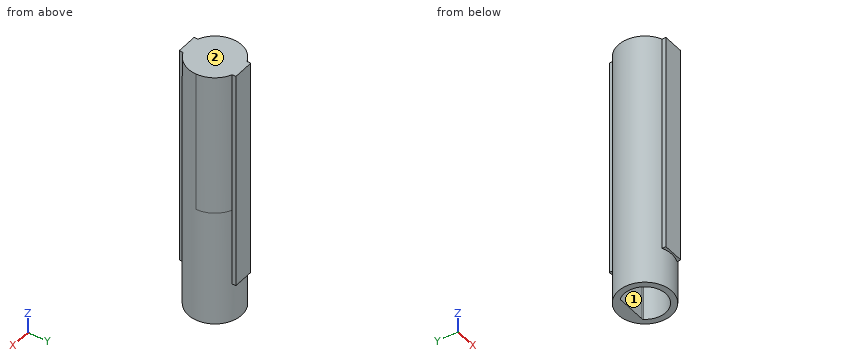
from build123d import *
from build123d.topology import SkipClean

# Parameters (mm, degrees)
SKETCH1_R                = 2
BOSS_EXTRUDE1_DEPTH      = 7
SKETCH3_R                = 2
SKETCH3_W                = 4.25
SKETCH3_H                = 1.5
BOSS_EXTRUDE3_DEPTH      = 4
BOSS_EXTRUDE4_START      = 4
BOSS_EXTRUDE4_DEPTH      = 4
BOSS_EXTRUDE5_START      = -8
BOSS_EXTRUDE5_DEPTH      = 8
CUT_EXTRUDE1_START       = -8
CUT_EXTRUDE1_DEPTH       = 8
CUT_EXTRUDE2_DEPTH       = 7
BOSS_EXTRUDE6_DEPTH      = 8
BOSS_EXTRUDE6_DEPTH_BACK = 3
SKETCH2_R                = 2.05
SKETCH2_R_2              = 2
BOSS_EXTRUDE7_START      = -8
BOSS_EXTRUDE7_DEPTH      = 8
BOSS_EXTRUDE8_DEPTH      = 9
BOSS_EXTRUDE8_DEPTH_BACK = 7
SKETCH11_R               = 2.05
BOSS_EXTRUDE9_DEPTH      = 9
FILLET1_R                = 0.1


with BuildPart() as part:
    # Sketch1 → Boss-Extrude1 (new body)
    with BuildSketch(Plane.XY):
        Circle(SKETCH1_R)
        with BuildLine():
            ThreePointArc((-1.5, 0), (-1.401258538, 0.535233135), (-1.118033989, 1))
            Line((-1.118033989, 1), (1.118033989, 1))
            ThreePointArc((1.118033989, 1), (1.401258538, 0.535233135), (1.5, 0))
            ThreePointArc((1.5, 0), (0, -1.5), (-1.5, 0))
        make_face(mode=Mode.SUBTRACT)
    extrude(amount=BOSS_EXTRUDE1_DEPTH)

    # Sketch3 → Boss-Extrude3 (add)
    with BuildSketch(Plane.XY.offset(7)):
        with Locations(Location((0, 0, 0), (0, 0, 157.975687163))):
            Circle(SKETCH3_R)
        Rectangle(SKETCH3_W, SKETCH3_H)
    extrude(amount=BOSS_EXTRUDE3_DEPTH)

    # Sketch4 → Boss-Extrude4 (add)
    with BuildSketch(Plane(origin=(0, 0, 7), x_dir=(-1, 0, 0), z_dir=(0, 0, -1)).offset(BOSS_EXTRUDE4_START)):
        with BuildLine():
            Line((-2.125, -0.75), (-1.854049622, -0.75))
            ThreePointArc((-1.854049622, -0.75), (-2, 0), (-1.854049622, 0.75))
            Line((-1.854049622, 0.75), (-2.125, 0.75))
            Line((-2.125, 0.75), (-2.125, -0.75))
        make_face()
        with BuildLine():
            Line((2.125, 0.75), (1.854049622, 0.75))
            ThreePointArc((1.854049622, 0.75), (2, 0), (1.854049622, -0.75))
            Line((1.854049622, -0.75), (2.125, -0.75))
            Line((2.125, -0.75), (2.125, 0.75))
        make_face()
    extrude(amount=-BOSS_EXTRUDE4_DEPTH)

    # Sketch6 → Boss-Extrude5 (add)
    with BuildSketch(Plane.XY.offset(11).offset(BOSS_EXTRUDE5_START)):
        with BuildLine():
            Line((-0.75, -1.854049622), (-0.75, -2.125))
            Line((-0.75, -2.125), (0.75, -2.125))
            Line((0.75, -2.125), (0.75, -1.854049622))
            ThreePointArc((0.75, -1.854049622), (0, -2), (-0.75, -1.854049622))
        make_face()
        with BuildLine():
            Line((0.75, 1.854049622), (0.75, 2.125))
            Line((0.75, 2.125), (-0.75, 2.125))
            Line((-0.75, 2.125), (-0.75, 1.854049622))
            ThreePointArc((-0.75, 1.854049622), (0, 2), (0.75, 1.854049622))
        make_face()
    extrude(amount=BOSS_EXTRUDE5_DEPTH)

    # Sketch7 → Cut-Extrude1 (cut)
    with SkipClean():  # the faces are left unmerged after this step: merging them gives an invalid solid
        with BuildSketch(Plane.XY.offset(11).offset(CUT_EXTRUDE1_START)):
            with BuildLine():
                Line((-2.125, -0.75), (-1.854049622, -0.75))
                ThreePointArc((-1.854049622, -0.75), (-2, 0), (-1.854049622, 0.75))
                Line((-1.854049622, 0.75), (-2.125, 0.75))
                Line((-2.125, 0.75), (-2.125, -0.75))
            make_face()
            with BuildLine():
                Line((1.854049622, -0.75), (2.125, -0.75))
                Line((2.125, -0.75), (2.125, 0.75))
                Line((2.125, 0.75), (1.854049622, 0.75))
                ThreePointArc((1.854049622, 0.75), (2, 0), (1.854049622, -0.75))
            make_face()
        extrude(amount=CUT_EXTRUDE1_DEPTH, mode=Mode.SUBTRACT)

    # Sketch8 → Cut-Extrude2 (cut)
    with SkipClean():  # the faces are left unmerged after this step: merging them gives an invalid solid
        with BuildSketch(Plane(origin=(0, 0, 0), x_dir=(-1, 0, 0), z_dir=(0, 0, -1))):
            with BuildLine():
                Line((-1.183215957, 1.15), (1.183215957, 1.15))
                ThreePointArc((1.183215957, 1.15), (0, -1.65), (-1.183215957, 1.15))
            make_face()
            with BuildLine():
                Line((-1.118033989, 1), (1.118033989, 1))
                ThreePointArc((1.118033989, 1), (0, -1.5), (-1.118033989, 1))
            make_face(mode=Mode.SUBTRACT)
        extrude(amount=-CUT_EXTRUDE2_DEPTH, mode=Mode.SUBTRACT)

    # Sketch2 → Boss-Extrude6 (add, two sides: drawn at the far end of the back side and taken through both)
    with BuildSketch(Plane.XY.offset(3).offset(-BOSS_EXTRUDE6_DEPTH_BACK)):
        Circle(SKETCH2_R)
        Circle(SKETCH2_R_2, mode=Mode.SUBTRACT)
    extrude(amount=BOSS_EXTRUDE6_DEPTH + BOSS_EXTRUDE6_DEPTH_BACK)

    # Sketch10 → Boss-Extrude7 (add)
    with BuildSketch(Plane(origin=(0, 0, 3), x_dir=(-1, 0, 0), z_dir=(0, 0, -1)).offset(BOSS_EXTRUDE7_START)):
        with BuildLine():
            Line((0.75, -1.907878403), (0.75, -2.125))
            Line((0.75, -2.125), (-0.75, -2.125))
            Line((-0.75, -2.125), (-0.75, -1.907878403))
            ThreePointArc((-0.75, -1.907878403), (-0.77506725, -1.897833174), (-0.8, -1.887458609))
            Line((-0.8, -1.887458609), (-0.8, -2.175))
            Line((-0.8, -2.175), (0.8, -2.175))
            Line((0.8, -2.175), (0.8, -1.887458609))
            ThreePointArc((0.8, -1.887458609), (0.77506725, -1.897833174), (0.75, -1.907878403))
        make_face()
        with BuildLine():
            Line((-0.8, 2.175), (-0.8, 1.887458609))
            ThreePointArc((-0.8, 1.887458609), (-0.77506725, 1.897833174), (-0.75, 1.907878403))
            Line((-0.75, 1.907878403), (-0.75, 2.125))
            Line((-0.75, 2.125), (0.75, 2.125))
            Line((0.75, 2.125), (0.75, 1.907878403))
            ThreePointArc((0.75, 1.907878403), (0.77506725, 1.897833174), (0.8, 1.887458609))
            Line((0.8, 1.887458609), (0.8, 2.175))
            Line((0.8, 2.175), (-0.8, 2.175))
        make_face()
    extrude(amount=BOSS_EXTRUDE7_DEPTH)

    # Sketch11 → Boss-Extrude8 (add, two sides: drawn at the far end of the back side and taken through both)
    with BuildSketch(Plane(origin=(0, 0, 0), x_dir=(-1, 0, 0), z_dir=(0, 0, -1)).offset(-BOSS_EXTRUDE8_DEPTH_BACK)):
        with Locations(Location((0, 0, 0), (0, 0, 112.969676572))):
            Circle(SKETCH11_R)
        with BuildLine():
            Line((-1.207269647, 1.05), (1.207269647, 1.05))
            ThreePointArc((1.207269647, 1.05), (0, -1.6), (-1.207269647, 1.05))
        make_face(mode=Mode.SUBTRACT)
    extrude(amount=BOSS_EXTRUDE8_DEPTH + BOSS_EXTRUDE8_DEPTH_BACK)

    # Sketch12 → Boss-Extrude9 (add)
    with BuildSketch(Plane(origin=(0, 0, 3), x_dir=(-1, 0, 0), z_dir=(0, 0, -1))):
        with BuildLine():
            Line((-0.8, 2.175), (-0.8, 1.887458609))
            ThreePointArc((-0.8, 1.887458609), (0, 2.05), (0.8, 1.887458609))
            Line((0.8, 1.887458609), (0.8, 2.175))
            Line((0.8, 2.175), (-0.8, 2.175))
        make_face()
        with BuildLine():
            Line((0.8, -2.175), (0.8, -1.887458609))
            ThreePointArc((0.8, -1.887458609), (0, -2.05), (-0.8, -1.887458609))
            Line((-0.8, -1.887458609), (-0.8, -2.175))
            Line((-0.8, -2.175), (0.8, -2.175))
        make_face()
    extrude(amount=BOSS_EXTRUDE9_DEPTH)

    # Fillet1
    fillet1_edges = [part.edges().sort_by_distance(p)[0] for p in [
        (1.207269647, 1.05, -4.5),
        (-1.207269647, 1.05, -4.5),
    ]]
    fillet(fillet1_edges, radius=FILLET1_R)


solid = part.part
Build history of the part. All positions in model axes, mm. Face numbers are marked on the shaded views. Round coordinates to 2 decimals unless told otherwise and drop trailing zeros. Write each loop counter-clockwise with the first axis right and the second up, starting at its lowest first coordinate (ties: lowest second). Pieces come first, ordered by that corner, then holes. Notation, with made-up numbers: (65.25, 41.25) - (115.25, 41.25) arc R19 ccw to (115.25, 53.25) - close; hole circle Ø3 at (68, -33.5). An arc over 180 degrees is marked (long way). One line per question, with ' | ' between items.
1. Drill centre lines: line 1 along X through (y, z) = (0, 2.5); line 2 along Y through (x, z) = (0, -0.75) (3 decimals); line 3 along Z through (x, y) = (-0.65, 0.35). Where is each one in solid material? Low to high. Write a range as from..to.
Results are:
line 1: -2.05..-1.6, 1.6..2.05 | line 2: -2.175..-1.6, 1.05..2.175 | line 3: 7..11
2. Mould opens along Y. For the marked faces 1 and 2 say: released by +Y, released by -Y, zero draft, split by the parting line, or undercut.
Results are:
face 1: undercut | face 2: zero draft
3. Band-saw the part on C-C, the plane z = 8.5. Write the cut outline in (x, y) (3 decimals), and give its area (3 significant figures).
Results are:
outline: (-0.8, -2.175) - (0.8, -2.175) - (0.8, -1.887) arc R2.05 ccw to (0.8, 1.887) - (0.8, 2.175) - (-0.8, 2.175) - (-0.8, 1.887) arc R2.05 ccw to (-0.8, -1.887) - close | area: 13.8 mm^2
4. Drop a flat-ended pin along its axis: pin 1 Ø1 at (x, y) = (-1, 0) entering from -Z. Give the stop position or say it passes through.
Results are:
pin 1: z = 7
5. Band-saw the part on B-B, the plane x = 0. Write the cut outline in (y, z) (3 decimals), and give its area (4 significant figures).
Results are:
outline: (-2.175, -6) - (-2.05, -6) - (-2.05, -9) - (-1.6, -9) - (-1.6, 7) - (1.05, 7) - (1.05, -9) - (2.05, -9) - (2.05, -6) - (2.175, -6) - (2.175, 11) - (-2.175, 11) - close | area: 43.85 mm^2
6. Band-saw the part on A-A, the plane z = 4.5. Write the cut outline in (x, y) (3 decimals).
Results are:
outline: (-0.8, -2.175) - (0.8, -2.175) - (0.8, -1.887) arc R2.05 ccw to (0.8, 1.887) - (0.8, 2.175) - (-0.8, 2.175) - (-0.8, 1.887) arc R2.05 ccw to (-0.8, -1.887) - close; hole (-1.238, 1.013) arc R1.6 ccw (long way) to (1.238, 1.013) arc R0.1 ccw to (1.161, 1.05) - (-1.161, 1.05) arc R0.1 ccw to start
7. Band-saw the part on D-D, the plane y = 1.55. Write the cut outline in (x, z).
Results are:
outline: (-1.34, -9) - (1.34, -9) - (1.34, 11) - (-1.34, 11) - close
